Geometry: final body of the model. Coordinates: model frame, mm. Face numbers are marked on the shaded views. A direction names the side the tool comes from. Coordinates: 2 decimals unless noted, no trailing zeros. Order: outer loops, then holes, each group sorted by start corner. A loop starts at its lowest first (then second) coordinate and runs counter-clockwise, first axis right, second up. Notation, with made-up numbers: M 43.25,-5.5 L 57.25,-5.5 A19 ccw 57.25,9.5 Z; hole C 38,0.25 d9. An arc over 180 degrees is marked long. Use CSV: the item, a comma, the result in double quotes. Start each with the question number.
Q1. Section query A-A, the plane z = 43.5. Output: boundary loops of the cut face in (x, y), and give its area (3 significant figures).
Q2. Section query B-B, the plane x = -110.75. Output: boundary loops of the cut face in (y, z), and give its area (3 significant figures).
Q3. Section query D-D, the plane x = -117.75. Output: boundary loops of the cut face in (y, z).
Q4. Access query for the marked faces 1 and 2. Directions: +Z, -Z, +X, -X, +Y, -Y. A direction counts if a zero-diameter tool reaches every point of the face in a straight line with its end or side. Return the directions, or none.
Q5. Mould query, pull axis Z, two halves, no side actions, for the marked faces 3, 4, 5 and 6. Classes: +Z half, -Z half, draft (parallel to the pull), parting line (faces both ways), or undercut.
Q6. Section query C-C, the plane y = 31.5. Output: boundary loops of the cut face in (x, z).
Q7. First-contact query: P1, Ø4, axis at x = -112, z = 28.5, coming from the +Y side; P2, Ø3.5, axis at x = -116.88, z = 43.5, coming from the -Y side; P3, Ø1, axis at y = 33.5, z = 16, coming from the +X side. Flat tips, straight axial feed; report the tip coordinate or a pass-through.
Q8. Ray query, probe 1 along X at (y, z) = (31.5, 43.5); probe 2 along Z at (x, y) = (-111, 33.25); probe 3 along Z at (x, y) = (-116.5, 31.75). Return the intervals inside material, ascending.
from build123d import *

# Parameters (mm, degrees)
ESQUISSE1_W             = 15
ESQUISSE1_H             = 3
BOSS_EXTRU_1_DEPTH      = 50
ESQUISSE2_R             = 1.6
ENL_V_MAT_EXTRU_1_DEPTH = 45
ESQUISSE3_W             = 15
ESQUISSE3_H             = 2.5
BOSS_EXTRU_2_DEPTH      = 15
ESQUISSE4_R             = 2.5
ENL_V_MAT_EXTRU_3_DEPTH = 65


with BuildPart() as part:
    # Esquisse1 → Boss.-Extru.1 (new body)
    with BuildSketch(Plane.XY):
        with Locations((-116.877940306, 30.735985997)):
            Rectangle(ESQUISSE1_W, ESQUISSE1_H)
    extrude(amount=BOSS_EXTRU_1_DEPTH)

    # Esquisse2 → Enlèv. mat.-Extru.1 (cut)
    with BuildSketch(Plane(origin=(0, 32.235985997, 0), x_dir=(1, 0, 0), z_dir=(0, 1, 0))):
        with Locations(Location((-116.877940306, -43.5, 0), (0, 0, 270))):
            Circle(ESQUISSE2_R)
        with Locations(Location((-116.877940306, -6.5, 0), (0, 0, 270))):
            Circle(ESQUISSE2_R)
    extrude(amount=-ENL_V_MAT_EXTRU_1_DEPTH, mode=Mode.SUBTRACT)

    # Esquisse3 → Boss.-Extru.2 (add)
    with BuildSketch(Plane(origin=(0, 32.235985997, 0), x_dir=(1, 0, 0), z_dir=(0, 1, 0))):
        with Locations((-116.877940306, -48.75)):
            Rectangle(ESQUISSE3_W, ESQUISSE3_H)
        with Locations((-116.877940306, -1.25)):
            Rectangle(ESQUISSE3_W, ESQUISSE3_H)
    extrude(amount=BOSS_EXTRU_2_DEPTH)

    # Esquisse4 → Enlèv. mat.-Extru.3 (cut)
    with BuildSketch(Plane.XY.offset(50)):
        with Locations((-116.877940306, 40.235985997)):
            Circle(ESQUISSE4_R)
    extrude(amount=-ENL_V_MAT_EXTRU_3_DEPTH, mode=Mode.SUBTRACT)


solid = part.part
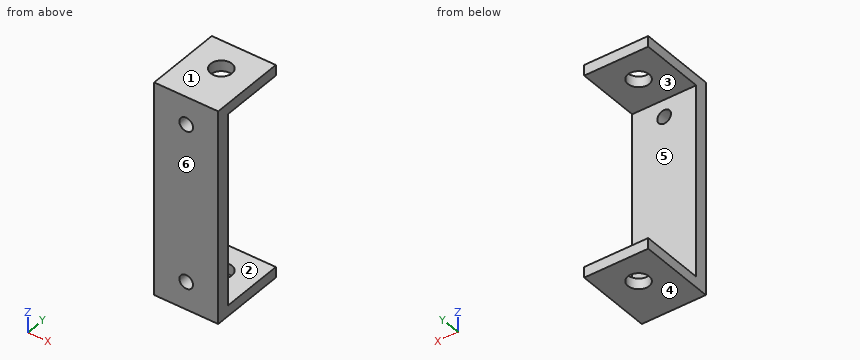
Responses:
1,outline,"M -124.38,29.24 L -118.48,29.24 L -118.48,32.24 L -124.38,32.24 Z; M -115.28,29.24 L -109.38,29.24 L -109.38,32.24 L -115.28,32.24 Z"
1,area,"35.4 mm²"
2,outline,"M 29.24,0 L 47.24,0 L 47.24,2.5 L 32.24,2.5 L 32.24,47.5 L 47.24,47.5 L 47.24,50 L 29.24,50 Z"
2,area,"225 mm²"
3,outline,"M 29.24,0 L 37.89,0 L 37.89,2.5 L 32.24,2.5 L 32.24,5.16 L 29.24,5.16 Z; M 29.24,7.84 L 32.24,7.84 L 32.24,42.16 L 29.24,42.16 Z; M 29.24,44.84 L 32.24,44.84 L 32.24,47.5 L 37.89,47.5 L 37.89,50 L 29.24,50 Z; M 42.58,0 L 47.24,0 L 47.24,2.5 L 42.58,2.5 Z; M 42.58,47.5 L 47.24,47.5 L 47.24,50 L 42.58,50 Z"
4,face 1,"+Z, +X, -X, +Y, -Y"
4,face 2,"+X, -X, +Y"
5,face 3,"undercut"
5,face 4,"-Z half"
5,face 5,"undercut"
5,face 6,"draft"
6,outline,"M -124.38,0 L -109.38,0 L -109.38,50 L -124.38,50 Z; hole C -116.88,6.5 d3.2; hole C -116.88,43.5 d3.2"
7,P1,"stops at y = 32.24"
7,P2,"stops at y = 29.24"
7,P3,"passes through"
8,probe 1,"x = -124.38 to -118.48, -115.28 to -109.38"
8,probe 2,"z = 0 to 2.5, 47.5 to 50"
8,probe 3,"z = 0 to 4.95, 8.05 to 41.95, 45.05 to 50"
